Autodesk Inventor part; units mm, degrees
ref_plane "YZ Plane" through (0, 0, 0) normal (1, 0, 0) x (0, 1, 0)
ref_plane "XZ Plane" through (0, 0, 0) normal (0, 1, 0) x (-1, 0, 0)
ref_plane "XY Plane" through (0, 0, 0) normal (0, 0, 1) x (1, 0, 0)
sketch "Sketch1" plane through (0, 0, 0) normal (1, 0, 0) x (0, 1, 0)
  line L0 (-15.5, 31.5) -> (15.5, 31.5)
  line L1 (15.5, 31.5) -> (15.5, -31.5)
  line L2 (15.5, -31.5) -> (-15.5, -31.5)
  line L3 (-15.5, -31.5) -> (-15.5, 31.5)
  line L4 (-15.5, 31.5) -> (15.5, -31.5) construction
  line L5 (15.5, 31.5) -> (-15.5, -31.5) construction
  circle A0 centre (5.5, 26.5) radius 1.6
  circle A1 centre (5.5, -26.5) radius 1.6
  circle A2 centre (-9.5, -26.5) radius 1.6
  circle A3 centre (-9.5, 26.5) radius 1.6
  circle A4 centre (0, 10.5) radius 6
  circle A5 centre (0, -10.5) radius 6
  point P0 (0, 0)
  point P1 (-9.5, 26.5)
  point P2 (5.5, -26.5)
  point P3 (-9.5, -16)
  dimension "d0" = 63
  dimension "d1" = 31
  dimension "d2" = 5
  dimension "d3" = 10
  dimension "d5" = 15
  dimension "d6" = 5
  dimension "d7" = 3.2
  dimension "d8" = 3.2
  dimension "d9" = 3.2
  dimension "d10" = 3.2
  dimension "d15" = 5
  dimension "d16" = 5
  dimension "d17" = 5
  dimension "d18" = 21
  dimension "d19" = 21
  dimension "d20" = 12
  dimension "d21" = 12
extrude "Extrusion1" add sketch "Sketch1" along normal blind 2 contours L0 L1 L2 L3 | A4 | A5
fillet "Fillet1" radius 2 4 edges at (1, 15.5, 31.5) (1, -15.5, 31.5) (1, -15.5, -31.5) (1, 15.5, -31.5)
sketch "Sketch2" plane through (2, 0, 0) normal (1, 0, 0) x (0, 0, -1)
  line L0 (21.5, -10.5) -> (-21.5, -10.5)
  line L1 (-21.5, -10.5) -> (-21.5, 10.5)
  line L2 (-21.5, 10.5) -> (21.5, 10.5)
  line L3 (21.5, 10.5) -> (21.5, -10.5)
  line L4 (21.5, -10.5) -> (-21.5, 10.5) construction
  line L5 (-21.5, -10.5) -> (21.5, 10.5) construction
  line L6 (29.5, 15.5) -> (-29.5, 15.5)
  line L7 (-29.5, -15.5) -> (29.5, -15.5)
  line L8 (31.5, -13.5) -> (31.5, 13.5)
  line L9 (-31.5, 13.5) -> (-31.5, -13.5)
  line L10 (-21.5, 10.5) -> (21.5, -10.5)
  line L11 (21.5, 10.5) -> (-21.5, -10.5)
  line L12 (-21.5, 7.5) -> (15.3571, -10.5)
  line L13 (-18.5, 10.5) -> (21.5, -9.0349)
  line L14 (0, 10.5) -> (0, 6.4862)
  line L15 (21.5, 7.5) -> (-15.3571, -10.5)
  line L16 (18.5, 10.5) -> (-21.5, -9.0349)
  point P0 (0, 0)
  point P1 (0, -3)
  point P2 (-15.3571, -10.5)
  point P3 (21.5, 7.5)
  point P4 (4.5714, -0.7674)
  point P5 (0, 1.4651)
  point P6 (18.5, 10.5)
  point P7 (-21.5, -9.0349)
  point P8 (-4.5714, -0.7674)
  dimension "d22" = 5
  dimension "d23" = 5
  dimension "d24" = 10
  dimension "d25" = 10
  dimension "d26" = 3
  dimension "d27" = 3
  dimension "d31" = 180
extrude "Extrusion2" cut sketch "Sketch2" against normal blind 2 contours L0 L15 L12 | L13 L15 L3 | L1 L12 L16 | L16 L13 L2
fillet "Fillet2" radius 2.5 12 edges at (1, 7.5, 21.5) (1, 10.5, 18.5) (1, 10.5, -18.5) (1, 7.5, -21.5) (1, -9.0349, -21.5) (1, -10.5, -15.3571) (1, -3, 0) (1, 1.4651, 0) (1, -0.7674, -4.5714) (1, -0.7674, 4.5714) (1, -10.5, 15.3571) (1, -9.0349, 21.5)
equation "\"d15\" = d2"
equation "\"d16\" = d6"
equation "\"d17\" = d6"
properties part number "2mm_double_for_pulley" material "アルミニウム 6061"
Work out the finished part from the listing and answer in its coordinate system (mm). A direction names the side the tool comes from. Round coordinates to 2 decimals unless told otherwise and drop trailing zeros. Loops run counter-clockwise (first coordinate to the right, second up) from the corner with the lowest first, then second, coordinate; pieces in that order, holes last. Notation, with made-up numbers: M 30.25,57 L 61.25,57 A15 cw 61.25,73 Z; hole C -4,70.5 d2. An arc over 180 degrees is marked long. One line per question, with ' | ' between items.
Q1. Find section B-B, the plane y = -9.5. Give the vertices of the cut face in (x, z).
Conclusion:
outline: M 0,-31.5 L 2,-31.5 L 2,-28.1 L 0,-28.1 Z; M 0,-24.9 L 2,-24.9 L 2,-6.54 L 0,-6.54 Z; M 0,6.54 L 2,6.54 L 2,24.9 L 0,24.9 Z; M 0,28.1 L 2,28.1 L 2,31.5 L 0,31.5 Z
Q2. Find section A-A, the plane z = 26.5. Give the vertices of the cut face in (x, y).
Conclusion:
outline: M 0,-15.5 L 2,-15.5 L 2,-11.1 L 0,-11.1 Z; M 0,-7.9 L 2,-7.9 L 2,3.9 L 0,3.9 Z; M 0,7.1 L 2,7.1 L 2,15.5 L 0,15.5 Z
Q3. A tool of negligible diameter and unlimited length cuts with its end or side. For faces 5 (the flat face through (1, 15.5, 0)), 6 (the cylindrical face through (0.99, 5.6, 20.35)), from which of +Z, -Z, +X, -X, +Y, -Y can it reach the whole face along a straight path? Write none if from no direction.
Conclusion:
face 5: +Z, -Z, +X, -X, +Y | face 6: +X, -X
Q4. Find section C-C, the plane z = 13.5. Give the vertices of the cut face in (x, y), then the cut area to 3 significant figures.
Conclusion:
outline: M 0,-15.5 L 2,-15.5 L 2,-5.13 L 0,-5.13 Z; M 0,3.59 L 2,3.59 L 2,15.5 L 0,15.5 Z | area: 44.6 mm2
Q5. The mould has two halves that part along Y. Classify faces 1 (the cylindrical face through (1.01, 14.9, -30.93)), 2 (the cylindrical face through (0.986, -8.609, 6.966)), 3 (the flat face through (1, 0, 31.5)), 4 (the flat face through (1, -15.5, 0)): +Y half, -Y half, draft (parallel to the pull), parting line (faces both ways), or undercut.
Conclusion:
face 1: +Y half | face 2: undercut | face 3: draft | face 4: -Y half
Q6. Consider line 1 along Z through (x, y) = (0.1, 1); line 2 along Z through (x, y) = (1.95, -9); line 3 along Z through (x, y) = (0.1, -8.5). Determine where each line is inside the solid, lowest interval first. Write a range as from..to.
Conclusion:
line 1: z = -31.5..-21.5, -8.5..8.5, 21.5..31.5 | line 2: z = -31.5..-28.02, -24.98..-6.83, 6.83..24.98, 28.02..31.5 | line 3: z = -31.5..-27.75, -25.25..-6.99, 6.99..25.25, 27.75..31.5
Q7. Find section D-D, the plane y = -1. Give the vertices of the cut face in (x, z), then the cut area to 3 significant figures.
Conclusion:
outline: M 0,-31.5 L 2,-31.5 L 2,-21.5 L 0,-21.5 Z; M 0,-7.78 L 2,-7.78 L 2,7.78 L 0,7.78 Z; M 0,21.5 L 2,21.5 L 2,31.5 L 0,31.5 Z | area: 71.1 mm2
